from build123d import *

# Parameters (mm, degrees)
SKETCH1_W                      = 156
SKETCH1_H                      = 84.5
BOSS_EXTRUDE1_DEPTH            = 12
CUT_EXTRUDE1_DEPTH             = 3
F_2_5_2_5_DIAMETER_HOLE1_D     = 2.5
F_2_5_2_5_DIAMETER_HOLE1_DEPTH = 10
F_6_1_6_1_DIAMETER_HOLE1_D     = 6.1
F_4_2_4_2_DIAMETER_HOLE1_D     = 4.2
F_4_2_4_2_DIAMETER_HOLE1_DEPTH = 8


with BuildPart() as part:
    # Sketch1 → Boss-Extrude1 (new body)
    with BuildSketch(Plane.XY.offset(12)):
        with Locations((0, -7.75)):
            Rectangle(SKETCH1_W, SKETCH1_H)
    extrude(amount=-BOSS_EXTRUDE1_DEPTH)

    # Sketch2 → Cut-Extrude1 (cut)
    with BuildSketch(Plane(origin=(0, 0, 0), x_dir=(-1, 0, 0), z_dir=(0, 0, -1))):
        with BuildLine():
            Line((-10.5, 24.003958007), (-10.5, 34.5))
            Line((-10.5, 34.5), (-17.2, 34.5))
            Line((-17.2, 34.5), (-17.2, 20))
            Line((-17.2, 20), (-16.924538398, 20))
            ThreePointArc((-16.924538398, 20), (13.85764217, -22.235236753), (-10.5, 24.003958007))
        make_face()
    extrude(amount=-CUT_EXTRUDE1_DEPTH, mode=Mode.SUBTRACT)

    # Ø2.5 (2.5) Diameter Hole1
    with Locations(Plane(origin=(78, 0, 0), x_dir=(0, 0, -1), z_dir=(1, 0, 0))):
        with Locations((-6, 0)):
            Hole(F_2_5_2_5_DIAMETER_HOLE1_D / 2, depth=F_2_5_2_5_DIAMETER_HOLE1_DEPTH)

    # Ø6.1 (6.1) Diameter Hole1 (through all)
    with Locations(Plane(origin=(0, 0, 0), x_dir=(-1, 0, 0), z_dir=(0, 0, -1))):
        with Locations((-55, -40), (55, -40)):
            Hole(F_6_1_6_1_DIAMETER_HOLE1_D / 2)

    # Ø4.2 (4.2) Diameter Hole1
    with Locations(Plane.XY.offset(12)):
        with Locations((47, 22.5), (-47, 22.5), (47, -22.5), (-47, -22.5)):
            Hole(F_4_2_4_2_DIAMETER_HOLE1_D / 2, depth=F_4_2_4_2_DIAMETER_HOLE1_DEPTH)


solid = part.part
Here's how the part is built. I have some questions about the finished solid (model axes, mm). A direction names the side the tool comes from. Coordinates: 2 decimals unless noted, no trailing zeros. Loops run counter-clockwise (first coordinate to the right, second up) from the corner with the lowest first, then second, coordinate; pieces in that order, holes last.
1. For P1, Ø3.5, axis at x = 47, y = 22.5, coming from the +Z side; P2, Ø0.8, axis at y = 0.5, z = 6, coming from the +X side; P3, Ø15.5, axis at x = -8, y = 12.5, coming from the -Z side, each with a flat end and sliding along its axis, tell me the tip position at first contact or that it passes through.
2. Imagine slicing it at B-B, the plane x = -15. Please give me the cut outline in (y, z), and give its area (3 significant figures).
3. Imagine slicing it at C-C, the plane y = 22.5. Please give me the cut outline in (x, z), and give its area (3 significant figures).
4. Imagine slicing it at A-A, the plane y = -40. Please give me the cut outline in (x, z).
5. Imagine slicing it at D-D, the plane x = 4.5. Please give me the cut outline in (y, z), and give its area (3 significant figures).
6. I need wall thicknesses on L1, parallel to Y at x = 47, z = 5.5; L2, parallel to Y at x = 55, z = 7; L3, parallel to Y at x = 0, z = 2.05. Which ranges of each line are inside material? Lowest first, please.
7. If we mould it in two halves opening along Y, with no side actions, what happens to faces 1 (the flat face through (17.2, 27, 1)), 2 (the flat face through (-1, -50, 6)), 3 (the cylindrical face through (45.87, -20.73, 7.94))? For each: pulls with the +Y half, pulls with the -Y half, needs draft (parallel to the pull), parting line crosses it, or undercut.
8. For faces 4 (the cylindrical face through (-12.91, -22.8, 1.48)), 5 (the flat face through (10.5, 29, 1)), 6 (the flat face through (47, -22, 4)), which set-ups out of +Z, -Z, +X, -X, +Y, -Y let a thin tool reach every point of the face, with its end or its side?
Taken from the geometry:
1. P1: stops at z = 4
1. P2: stops at x = 68
1. P3: stops at z = 3
2. outline: (-50, 0) - (-21.48, 0) - (-21.48, 3) - (21.48, 3) - (21.48, 0) - (34.5, 0) - (34.5, 12) - (-50, 12) - close
2. area: 885 mm2
3. outline: (-78, 0) - (-13.42, 0) - (-13.42, 3) - (17.2, 3) - (17.2, 0) - (78, 0) - (78, 12) - (49.1, 12) - (49.1, 4) - (44.9, 4) - (44.9, 12) - (-44.9, 12) - (-44.9, 4) - (-49.1, 4) - (-49.1, 12) - (-78, 12) - close
3. area: 1,710 mm2
4. outline: (-78, 0) - (-58.05, 0) - (-58.05, 12) - (-78, 12) - close; (-51.95, 0) - (51.95, 0) - (51.95, 12) - (-51.95, 12) - close; (58.05, 0) - (78, 0) - (78, 12) - (58.05, 12) - close
5. outline: (-50, 0) - (-25.81, 0) - (-25.81, 3) - (25.81, 3) - (25.81, 0) - (34.5, 0) - (34.5, 12) - (-50, 12) - close
5. area: 859 mm2
6. L1: y = -50 to -24.6, -20.4 to 20.4, 24.6 to 34.5
6. L2: y = -50 to -43.05, -36.95 to 34.5
6. L3: y = -50 to -26.2, 26.2 to 34.5
7. face 1: needs draft
7. face 2: pulls with the -Y half
7. face 3: undercut
8. face 4: -Z
8. face 5: -Z, +Y
8. face 6: +Z
